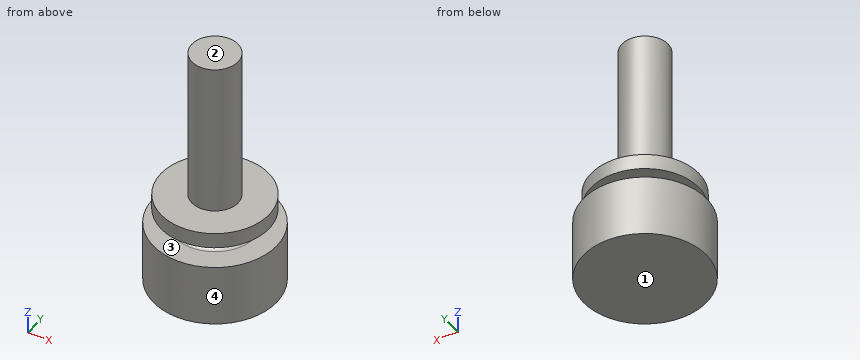
Autodesk Inventor part; units mm, degrees
ref_plane "YZ Plane" through (0, 0, 0) normal (1, 0, 0) x (0, 1, 0)
ref_plane "XZ Plane" through (0, 0, 0) normal (0, 1, 0) x (-1, 0, 0)
ref_plane "XY Plane" through (0, 0, 0) normal (0, 0, 1) x (1, 0, 0)
sketch "スケッチ1" plane through (0, 0, 0) normal (0, 1, 0) x (-1, 0, 0)
  line L0 (0, 0) -> (0, 16)
  line L1 (0, 0) -> (4, 0)
  line L2 (4, 0) -> (4, 4)
  line L3 (4, 4) -> (2.6, 4)
  line L4 (2.6, 4) -> (2.6, 5) construction
  line L5 (2.6, 5) -> (3.5, 5)
  line L6 (3.5, 5) -> (3.5, 6)
  line L7 (3.5, 6) -> (1.5, 6)
  line L8 (1.5, 6) -> (1.5, 16)
  line L9 (1.5, 16) -> (0, 16)
  arc A0 (2.6, 5) -> (2.6, 4) centre (2.6, 4.5) ccw
  line L10 (2.6, 4.5) -> (2.1, 4.5) construction
  dimension "d4" = 1
  dimension "d5" = 6
  dimension "d7" = 4
  dimension "d8" = 10
  dimension "d11" = 2.1
  dimension "d12" = 3
  dimension "d13" = 8
  dimension "d14" = 7
revolve "回転1" add sketch "スケッチ1" angle 360 about axis through (0, 0, 0) along (0, 0, 1)
thread "ねじ1"
properties part number "SPNFL-BRN-M3-10" material "ステンレス鋼 AISI 304"
For this review, take the finished solid that the model builds, in its own axes (mm). Face numbers are marked on the shaded views. Round coordinates to 2 decimals unless told otherwise and drop trailing zeros. Loops run counter-clockwise (first coordinate to the right, second up) from the corner with the lowest first, then second, coordinate; pieces in that order, holes last.
Q1. Insertion check: pin 1 Ø3 at (x, z) = (-0.5, 8) entering from +Y; pin 2 Ø4 at (y, z) = (1.5, 13) entering from -X; pin 3 Ø1.5 at (y, z) = (0.5, 8.5) entering from +X. Each pin has a flat end and moves straight along its axis. Give the tip position at first contact, or say it passes through.
Result sheet:
pin 1: stops at y = 1.5
pin 2: stops at x = -1.5
pin 3: stops at x = 1.5
Q2. Add section A-A on x = 0. Write out the cut boundary in (y, z), plus the area to 3 significant figures.
Result sheet:
outline: (-4, 0) - (4, 0) - (4, 4) - (2.6, 4) arc R0.5 cw to (2.6, 5) - (3.5, 5) - (3.5, 6) - (1.5, 6) - (1.5, 16) - (-1.5, 16) - (-1.5, 6) - (-3.5, 6) - (-3.5, 5) - (-2.6, 5) arc R0.5 cw to (-2.6, 4) - (-4, 4) - close
area: 73.4 mm2
Q3. Add section D-D on z = 14.75. Write out the cut boundary in (x, y), plus the area to 3 significant figures.
Result sheet:
outline: circle Ø3 at (0, 0)
area: 7.07 mm2
Q4. To check wall thickness, follow line 1 along Z through (x, y) = (-2.75, -0.5); line 2 along Y through (x, z) = (0, 15); line 3 along Z through (x, y) = (0.5, 3.75). State the ranges of each line that lie inside material, in increasing order.
Result sheet:
line 1: z = 0 to 4, 5 to 6
line 2: y = -1.5 to 1.5
line 3: z = 0 to 4
Q5. Mouldability with a two-part tool opening along Z and no side actions: class the marked faces 1, 2, 3 and 4 as +Z half, -Z half, draft (parallel to the pull), parting line (faces both ways), or undercut.
Result sheet:
face 1: -Z half
face 2: +Z half
face 3: undercut
face 4: draft
Q6. Add section B-B on x = 3. Write out the cut boundary in (y, z).
Result sheet:
outline: (-2.65, 0) - (2.65, 0) - (2.65, 4) - (-2.65, 4) - close; (-1.8, 5) - (1.8, 5) - (1.8, 6) - (-1.8, 6) - close
